The drawing under review shows one solid part. Ordinate dimensions are in mm from its lowest x, y, z. A direction names the side the tool comes from. Round coordinates to 2 decimals unless told otherwise and drop trailing zeros. Write each loop counter-clockwise with the first axis right and the second up, starting at its lowest first coordinate (ties: lowest second). Pieces come first, ordered by that corner, then holes. Notation, with made-up numbers: (-20.75, -12) -> (-6.75, -12) arc R28 cw to (-6.75, 6) -> close; hole circle Ø3 at (-16.75, 72). An arc over 180 degrees is marked (long way). Write item = value, one per line. Start each with the question number.
Item 1: Machinability: for the marked faces 1 and 2, which of the approach directions +Z, -Z, +X, -X, +Y, -Y give a long, thin tool a straight path to every point of the face, cutting with its end or side? Answer none if there is none.
Item 2: For pin 1 Ø4 at (x, z) = (56.15, 53.63) entering from -Y; pin 2 Ø2 at (x, y) = (61, 9.5) entering from +Z; pin 3 Ø2 at (y, z) = (5.5, 9) entering from -X (3 decimals); pin 4 Ø8 at (y, z) = (5, 35) entering from +X (3 decimals), all flat-tipped, find the tip position at first contact; note any pin that passes through.
Item 3: Mouldability with a two-part tool opening along Z and no side actions: class the marked faces 3, 4 and 5 as released by +Z, released by -Z, zero draft, split by the parting line, or undercut.
Item 4: Add section B-B, the plane y = 3.5. State the section outline as (x, z) points (1 decimal), then the cut area to 3 significant figures.
Item 5: To check wall thickness, follow L1, parallel to Z at x = 5.5, y = 12; L2, parallel to Z at x = 35.5, y = 7 (1 decimal); L3, parallel to X at y = 3.75, z = 45.5 (1 decimal). State the ranges of each line that lie inside material, in increasing order.
Item 6: Add section A-A, the plane z = 5.45. State the section outline as (x, y) points, then the cut area to 3 significant figures.
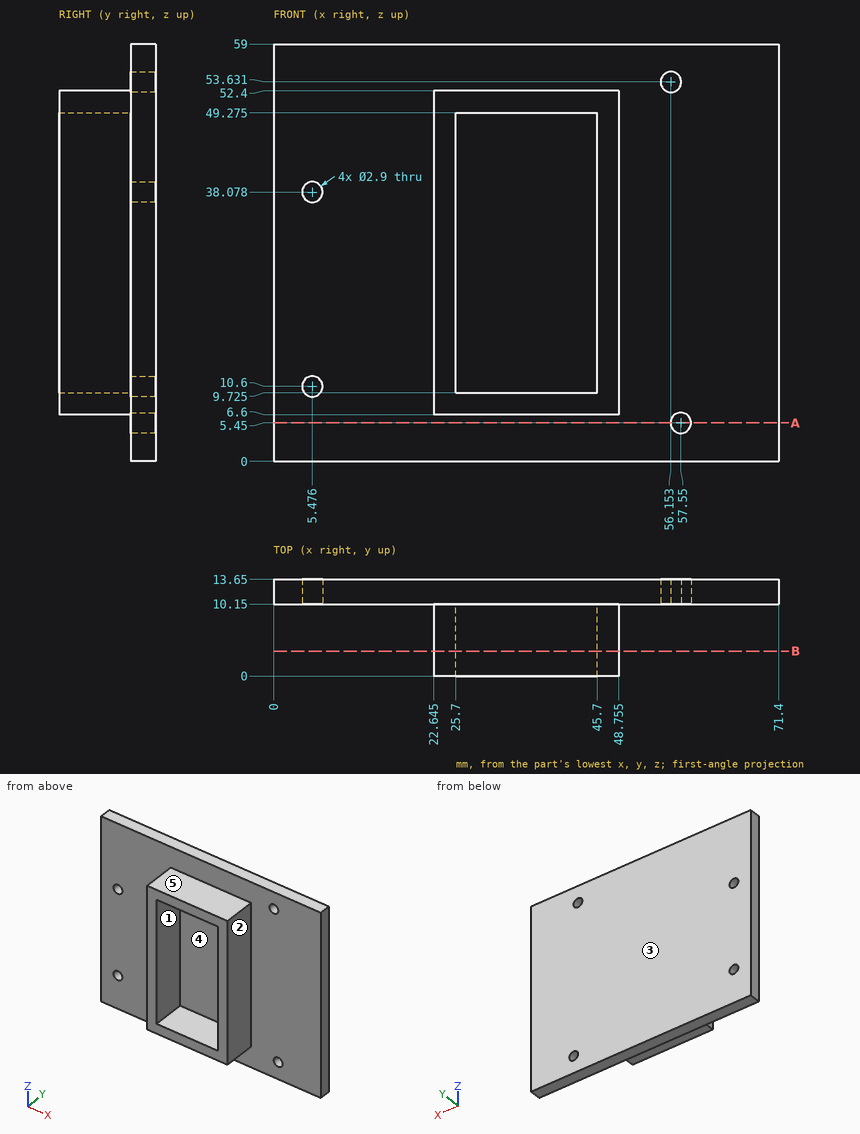
Result set:
q1.face_1 = -Y
q1.face_2 = +Z, -Z, +X, -Y
q2.pin_1 = 10.15
q2.pin_2 = 59
q2.pin_3 = 22.645
q2.pin_4 = 48.755
q3.face_3 = zero draft
q3.face_4 = undercut
q3.face_5 = released by +Z
q4.outline = (22.6, 6.6) -> (48.8, 6.6) -> (48.8, 52.4) -> (22.6, 52.4) -> close; hole (25.7, 9.7) -> (45.7, 9.7) -> (45.7, 49.3) -> (25.7, 49.3) -> close
q4.area = 405 mm²
q5.L1 = 0 to 9.15, 12.05 to 36.63, 39.53 to 59
q5.L2 = 6.6 to 9.7, 49.3 to 52.4
q5.L3 = 22.6 to 25.7, 45.7 to 48.8
q6.outline = (0, 10.15) -> (56.1, 10.15) -> (56.1, 13.65) -> (0, 13.65) -> close; (59, 10.15) -> (71.4, 10.15) -> (71.4, 13.65) -> (59, 13.65) -> close
q6.area = 240 mm²
